from build123d import *

# Parameters (mm, degrees)
SKETCH_1_W               = 625
SKETCH_1_H               = 470
SKETCH_1_W_2             = 571
SKETCH_1_H_2             = 416
EXTRUDE_1_DEPTH          = 4
FILLET_1_R               = 15
CUT_EXTRUDE_2_DEPTH      = 392.020779499
CUT_EXTRUDE_2_DEPTH_BACK = 392.020779499
SKETCH_3_R               = 3
SKETCH_4_R               = 3
CUT_EXTRUDE_3_DEPTH      = 392.082152495


with BuildPart() as part:
    # Эскиз1 → Бобышка-Вытянуть1 (new, symmetric)
    with BuildSketch(Plane(origin=(0, 0, 0), x_dir=(1, 0, 0), z_dir=(0, 1, 0))):
        Rectangle(SKETCH_1_W, SKETCH_1_H)
        Rectangle(SKETCH_1_W_2, SKETCH_1_H_2, mode=Mode.SUBTRACT)
    extrude(amount=EXTRUDE_1_DEPTH, both=True)

    # Скругление1
    fillet_1_edges = [part.edges().sort_by_distance(p)[0] for p in [
        (-312.5, 0, -235),
        (312.5, 0, -235),
        (312.5, 0, 235),
        (-312.5, 0, 235),
    ]]
    fillet(fillet_1_edges, radius=FILLET_1_R)

    # Эскиз3 → Вырез-Вытянуть2 (cut, two sides: drawn at the far end of the back side and taken through both)
    with BuildSketch(Plane(origin=(0, 0, 0), x_dir=(0, 0, -1), z_dir=(1, 0, 0)).offset(-CUT_EXTRUDE_2_DEPTH_BACK)):
        Circle(SKETCH_3_R)
    extrude(amount=CUT_EXTRUDE_2_DEPTH + CUT_EXTRUDE_2_DEPTH_BACK, mode=Mode.SUBTRACT)

    # Эскиз4 → Вырез-Вытянуть3 (cut, through all)
    with BuildSketch(Plane(origin=(0, 4, 0), x_dir=(1, 0, 0), z_dir=(0, 1, 0))):
        with Locations(Location((-299, 4, 0), (0, 0, 270))):
            Circle(SKETCH_4_R)
        with Locations(Location((299, 4, 0), (0, 0, 270))):
            Circle(SKETCH_4_R)
    extrude(amount=-CUT_EXTRUDE_3_DEPTH, mode=Mode.SUBTRACT)


solid = part.part
Design review of the part built by this model. Coordinates are the model's own, in mm. Coordinates: 2 decimals unless noted, no trailing zeros. Order: outer loops, then holes, each group sorted by start corner. A loop starts at its lowest first (then second) coordinate and runs counter-clockwise, first axis right, second up.
Item 1: Take a section at C-C, the plane y = 0. Write out the cut boundary in (x, z), then the cut area to 3 significant figures.
Item 2: For line 1 (X direction, y = 2.75, z = -4); line 2 (X direction, y = 0.25, z = 24); line 3 (Z direction, x = 262.5, y = -3.5), list the stretches that pass through material, from the lowest coordinate up.
Item 3: For pin 1 Ø9.5 at (x, z) = (299, -4) entering from -Y, flat-tipped, find the tip position at first contact; note if it passes through.
Item 4: Take a section at B-B, the plane x = 233. Write out the cut boundary in (y, z).
Item 5: Take a section at A-A, the plane z = 154.5. Write out the cut boundary in (x, y), then the cut area to 3 significant figures.
The answers:
1. outline: (-312.5, -220) arc R15 ccw to (-297.5, -235) - (297.5, -235) arc R15 ccw to (312.5, -220) - (312.5, -3) - (301.83, -3) arc R3 cw (long way) to (296.17, -3) - (285.5, -3) - (285.5, -208) - (-285.5, -208) - (-285.5, -3) - (-296.17, -3) arc R3 cw (long way) to (-301.83, -3) - (-312.5, -3) - close; (-312.5, 3) - (-285.5, 3) - (-285.5, 208) - (285.5, 208) - (285.5, 3) - (312.5, 3) - (312.5, 220) arc R15 ccw to (297.5, 235) - (-297.5, 235) arc R15 ccw to (-312.5, 220) - close
1. area: 55,700 mm2
2. line 1: x = -312.5 to -302, -296 to -285.5, 285.5 to 296, 302 to 312.5
2. line 2: x = -312.5 to -285.5, 285.5 to 312.5
2. line 3: z = -235 to -208, 208 to 235
3. pin 1: stops at y = -4
4. outline: (-4, -235) - (4, -235) - (4, -208) - (-4, -208) - close; (-4, 208) - (4, 208) - (4, 235) - (-4, 235) - close
5. outline: (-312.5, -4) - (-285.5, -4) - (-285.5, 4) - (-312.5, 4) - close; (285.5, -4) - (312.5, -4) - (312.5, 4) - (285.5, 4) - close
5. area: 432 mm2
